Read the model definition and answer for the solid it produces. Units are mm, in the model's axes. A direction names the side the tool comes from. Round coordinates to 2 decimals unless told otherwise and drop trailing zeros. Order: outer loops, then holes, each group sorted by start corner. A loop starts at its lowest first (then second) coordinate and runs counter-clockwise, first axis right, second up.
from build123d import *

# Parameters (mm, degrees)
F1_DEPTH = 6
F2_R     = 10
F3_W     = 30
F3_H     = 11
F4_DEPTH = 6
F5_R     = 1.5
F6_DEPTH = 25


with BuildPart() as f1:
    # F0 (on Top) → F1 (new body)
    with BuildSketch(Plane.XY):
        Polygon((120, 17.5), (-150, 17.5), (-150, -17.5), (120, -17.5), (120, -8.5), (0, -8.5), (0, -6.5), (150, -6.5), (150, 4.5), (0, 4.5), (0, 6.5), (120, 6.5), align=None)
    extrude(amount=F1_DEPTH)

    # F2
    f2_edges = [f1.edges().sort_by_distance(p)[0] for p in [
        (-150, -17.5, 3),
        (-150, 17.5, 3),
    ]]
    fillet(f2_edges, radius=F2_R)

    # F3 (on face) → F4 (join)
    with BuildSketch(Plane.XY.offset(6)):
        with Locations((135, -1)):
            Rectangle(F3_W, F3_H)
    extrude(amount=F4_DEPTH)

    # F5 (on face) → F6 (cut)
    with BuildSketch(Plane.XZ.offset(6.5)):
        with Locations((139.5, 6)):
            Circle(F5_R)
    extrude(amount=-F6_DEPTH, mode=Mode.SUBTRACT)


solid = f1.part
Q1. Straight lines are drawn through the part: probe 1 along Z at (x, y) = (139.5, 0); probe 2 along Z at (x, y) = (-36, 5); probe 3 along Y at (x, z) = (131, 2.75). For each, find the intervals that lie inside material, in ascending order.
Outcome:
probe 1: z = 0 to 4.5, 7.5 to 12
probe 2: z = 0 to 6
probe 3: y = -6.5 to 4.5
Q2. A cutting plane is placed at C-C, the plane y = -14. Give the vertices of the cut face in (x, z), plus the area to 3 significant figures.
Outcome:
outline: (-147.6, 0) - (120, 0) - (120, 6) - (-147.6, 6) - close
area: 1,610 mm2
Q3. A cutting plane is placed at B-B, the plane x = -98. Give the vertices of the cut face in (y, z).
Outcome:
outline: (-17.5, 0) - (17.5, 0) - (17.5, 6) - (-17.5, 6) - close
Q4. A cutting plane is placed at A-A, the plane x = 58. Give the vertices of the cut face in (y, z), plus the area to 3 significant figures.
Outcome:
outline: (-17.5, 0) - (-8.5, 0) - (-8.5, 6) - (-17.5, 6) - close; (-6.5, 0) - (4.5, 0) - (4.5, 6) - (-6.5, 6) - close; (6.5, 0) - (17.5, 0) - (17.5, 6) - (6.5, 6) - close
area: 186 mm2
Q5. For faces 4 (the face through (59, 6.5, 3)), 5 (the face through (-17, 0, 6)), 6 (the face through (120, 12, 3)), 7 (the face through (120, -13, 3)), determine the directions among +Z, -Z, +X, -X, +Y, -Y from which every point of the face is accessible in a straight line to the end or side of a thin tool.
Outcome:
face 4: +Z, -Z, +X
face 5: +Z, -X, +Y, -Y
face 6: +Z, -Z, +X, +Y
face 7: +Z, -Z, +X, -Y
Q6. Flat-ended cylindrical pins translate along their axes: pin 1 (3 mm diameter, centred on y = 1.5, z = 9.5, fed in from -X); pin 2 (17.5 mm diameter, centred on x = -78.5, y = -3.5, fed in from +Z); pin 3 (1.6 mm diameter, centred on y = -7.5, z = 1.5, fed in from +X). Find the tip coordinate at first contact, or state that the pin passes through.
Outcome:
pin 1: stops at x = 120
pin 2: stops at z = 6
pin 3: stops at x = 0
Q7. For a pull along Y with two mould halves and no side action, classify faces 1 (the face through (-8, 17.5, 3)), 2 (the face through (74, -6.5, 5)), 3 (the face through (-12, -17.5, 3)) as released by +Y, released by -Y, zero draft, split by the parting line, or undercut.
Outcome:
face 1: released by +Y
face 2: undercut
face 3: released by -Y
